For this review, take the finished solid that the model builds, in its own axes (mm). Coordinates: 2 decimals unless noted, no trailing zeros. Order: outer loops, then holes, each group sorted by start corner. A loop starts at its lowest first (then second) coordinate and runs counter-clockwise, first axis right, second up. Notation, with made-up numbers: M -24.75,23.5 L 2.25,23.5 A30 cw 2.25,58.5 Z; hole C 7,34.25 d5. An arc over 180 degrees is marked long. Use CSV: the item, a comma, the result in double quotes.
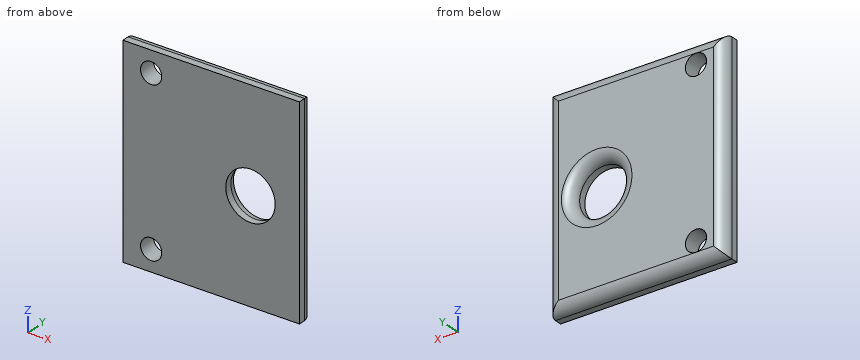
Autodesk Inventor part; units mm, degrees
ref_plane "YZ Plane" through (0, 0, 0) normal (1, 0, 0) x (0, 1, 0)
ref_plane "XZ Plane" through (0, 0, 0) normal (0, 1, 0) x (-1, 0, 0)
ref_plane "XY Plane" through (0, 0, 0) normal (0, 0, 1) x (1, 0, 0)
sketch "Эскиз1" plane through (0, 0, 0) normal (0, 1, 0) x (-1, 0, 0)
  line L0 (6.8605, 9.6174) -> (-18.1395, 9.6174)
  line L1 (-18.1395, 9.6174) -> (-18.1395, -19.3826)
  line L2 (-18.1395, -19.3826) -> (6.8605, -19.3826)
  line L3 (6.8605, -19.3826) -> (6.8605, 9.6174)
  circle A0 centre (2.8605, 6.6174) radius 1.5
  circle A1 centre (2.8605, -16.3826) radius 1.5
  circle A2 centre (-11.2073, -4.8826) radius 3.5
  point P0 (0, 0)
  dimension "d0" = 3
  dimension "d1" = 3
  dimension "d2" = 23
  dimension "d3" = 3
  dimension "d4" = 3
  dimension "d5" = 25
  dimension "d6" = 4
  dimension "d7" = 7
extrude "Выдавливание1" add sketch "Эскиз1" along normal blind 2.5
fillet "Сопряжение1" radius 1.5 1 edges at (14.7073, 2.5, -4.8826)
fillet "Сопряжение2" radius 1.5 4 edges at (5.6395, 2.5, 9.6174) (18.1395, 2.5, -4.8826) (5.6395, 2.5, -19.3826) (-6.8605, 2.5, -4.8826)
Item 1: Add section A-A on x = -3. State how many separate pieces and enclosed holes the cut face has, and give its area (3 significant figures).
Solutions:
separate pieces,"3"
enclosed holes,"0"
area,"56.6 mm^2"
Item 2: Add section C-C on z = -12.75. State the section outline as (x, y) points.
Solutions:
outline,"M -6.86,0 L 18.14,0 L 18.14,1 A1.5 ccw 16.64,2.5 L -5.36,2.5 A1.5 ccw -6.86,1 Z"
Item 3: Add section D-D on y = 2.1. State the section outline as (x, z) points.
Solutions:
outline,"M -6.38,-18.9 L 17.66,-18.9 L 17.66,9.14 L -6.38,9.14 Z; hole C -2.86,-16.38 d3; hole C -2.86,6.62 d3; hole C 11.21,-4.88 d7.96"
Item 4: Clearance check with a flat-ended pin moving along its axis: pin 1 Ø1.8 at (x, z) = (-2.86, 6.62) entering from +Y. State where the tip first meets the part, or that it passes through.
Solutions:
pin 1,"through"
Item 5: Add section B-B on y = 0.45. State the section outline as (x, z) points.
Solutions:
outline,"M -6.86,-19.38 L 18.14,-19.38 L 18.14,9.62 L -6.86,9.62 Z; hole C -2.86,-16.38 d3; hole C -2.86,6.62 d3; hole C 11.21,-4.88 d7"
Item 6: To check wall thickness, follow line 1 along X through (y, z) = (0.55, -2.25); line 2 along X through (y, z) = (0.8, -16.75); line 3 along Z through (x, y) = (-2.75, 2.2). State the ranges of each line that lie inside material, in increasing order. Write a range as [from, to].
Solutions:
line 1,"[-6.86, 8.9], [13.51, 18.14]"
line 2,"[-6.86, -4.31], [-1.41, 18.14]"
line 3,"[-18.78, -17.88], [-14.89, 5.12], [8.11, 9.02]"
